from build123d import *

# Parameters (mm, degrees)
SKETCH016_W     = 89
SKETCH016_H     = 89
SKETCH016_R     = 8.5
SKETCH016_R_2   = 2
PAD012_DEPTH    = 4.7
SKETCH021_R     = 2
POCKET003_DEPTH = 256.606458


with BuildPart() as part:
    # Sketch016 → Pad012 (new body)
    with BuildSketch(Plane.XY):
        Rectangle(SKETCH016_W, SKETCH016_H)
        with Locations((0, -22.5)):
            Circle(SKETCH016_R, mode=Mode.SUBTRACT)
        with Locations((-22, -22.5)):
            Circle(SKETCH016_R_2, mode=Mode.SUBTRACT)
        with Locations((22, -22.5)):
            Circle(SKETCH016_R_2, mode=Mode.SUBTRACT)
    extrude(amount=PAD012_DEPTH)

    # Sketch021 (on Face9 of Pad012) → Pocket003 (cut, through all)
    with BuildSketch(Plane.XY.offset(4.7)):
        with Locations((-27, 29.1)):
            Circle(SKETCH021_R)
    pocket003 = extrude(amount=-POCKET003_DEPTH, mode=Mode.SUBTRACT)

    # Mirrored002: Pocket003 across Sketch021 V_Axis
    add(pocket003.mirror(Plane(origin=(0, 0, 4.7), x_dir=(0, 0, 1), z_dir=(1, 0, 0))), mode=Mode.SUBTRACT)


with BuildPart() as part_1:
    # Body013 placement: moved
    add(part.part.moved(Location((0, 0, 99))))


with BuildPart() as part_2:
    # Clone006 placement: moved
    add(part_1.part.moved(Location((0, 0, -99))))


with BuildPart() as part_3:
    # Body019 placement: moved
    add(part_2.part.moved(Location((535, 6.5, 0))))


solid = part_3.part
Input: part model. Units: mm. Frame: model coordinates. Round coordinates to 2 decimals unless told otherwise and drop trailing zeros. Write each loop counter-clockwise with the first axis right and the second up, starting at its lowest first coordinate (ties: lowest second). Pieces come first, ordered by that corner, then holes.
1) Cut plane C-C (y = 35.6). Return the cut outline in (x, z).
2) Cut plane B-B (z = 3.85). Return the cut outline in (x, y).
3) Draft query along X for faces 1 (the cylindrical face through (506.002, 35.688, 2.383)), 2 (the flat face through (490.5, 6, 2)), 3 (the cylindrical face through (511, -16, 2)), 4 (the flat face through (534, 7, 4.7)). Return one class per face: pulls with the +X half, pulls with the -X half, needs draft (parallel to the pull), parting line crosses it, or undercut.
4) Cut plane A-A (x = 535). Return the cut outline in (y, z), then the cut area to 3 significant figures.
5) Cut plane D-D (x = 513). Return the cut outline in (y, z), then the cut area to 4 significant figures.
6) Ray query, L1, parallel to Y at x = 508, z = 1; L2, parallel to Y at x = 535, z = 3.3; L3, parallel to X at y = -21.5, z = 0.3. Return the intervals inside material, ascending.
7) Contact query for a flat-ended pin moving along its axis: P1, Ø3.5, axis at x = 562, y = 35.6, coming from the -Z side. Output: stop coordinate, or through.
Geometry says:
1. outline: (490.5, 0) - (506, 0) - (506, 4.7) - (490.5, 4.7) - close; (510, 0) - (560, 0) - (560, 4.7) - (510, 4.7) - close; (564, 0) - (579.5, 0) - (579.5, 4.7) - (564, 4.7) - close
2. outline: (490.5, -38) - (579.5, -38) - (579.5, 51) - (490.5, 51) - close; hole circle Ø4 at (508, 35.6); hole circle Ø4 at (513, -16); hole circle Ø17 at (535, -16); hole circle Ø4 at (557, -16); hole circle Ø4 at (562, 35.6)
3. face 1: undercut
3. face 2: pulls with the -X half
3. face 3: undercut
3. face 4: needs draft
4. outline: (-38, 0) - (-24.5, 0) - (-24.5, 4.7) - (-38, 4.7) - close; (-7.5, 0) - (51, 0) - (51, 4.7) - (-7.5, 4.7) - close
4. area: 338 mm2
5. outline: (-38, 0) - (-18, 0) - (-18, 4.7) - (-38, 4.7) - close; (-14, 0) - (51, 0) - (51, 4.7) - (-14, 4.7) - close
5. area: 399.5 mm2
6. L1: y = -38 to 33.6, 37.6 to 51
6. L2: y = -38 to -24.5, -7.5 to 51
6. L3: x = 490.5 to 528.52, 541.48 to 579.5
7. P1: passes through
